Autodesk Inventor part; units mm, degrees
ref_plane "YZ Plane" through (0, 0, 0) normal (1, 0, 0) x (0, 1, 0)
ref_plane "XZ Plane" through (0, 0, 0) normal (0, 1, 0) x (-1, 0, 0)
ref_plane "XY Plane" through (0, 0, 0) normal (0, 0, 1) x (1, 0, 0)
sketch "Boceto1" plane through (0, 0, 0) normal (0, 1, 0) x (-1, 0, 0)
  circle A0 centre (0, 0) radius 26
  circle A1 centre (0, 0) radius 32
  line L0 (0, 40) -> (32, 40)
  line L1 (32, 40) -> (32, -40)
  line L2 (32, -40) -> (0, -40)
  line L3 (0, -40) -> (0, 40)
  dimension "d0" = 52
  dimension "d1" = 64
  dimension "d2" = 40
  dimension "d3" = 80
  dimension "d4" = 32
  dimension "d5" = 32
extrude "Extrusión1" add sketch "Boceto1" along normal blind 67
sketch "Boceto2" plane through (0, 67, 0) normal (0, 1, 0) x (1, 0, 0)
  circle A0 centre (0, 0) radius 26
  dimension "d8" = 52
hole "Agujero1" at (0, 67, 0) direction (0, -1, 0) diameter 52 depth 60
sketch "Boceto3" plane through (0, 0, 0) normal (0, -1, 0) x (1, 0, 0)
  circle A0 centre (0, 0) radius 13
  dimension "d16" = 26
hole "Agujero2" at (0, 0, 0) direction (0, 1, 0) diameter 26 depth 60
sketch "Boceto4" plane through (0, 0, 0) normal (0, -1, 0) x (1, 0, 0)
  circle A0 centre (0, 0) radius 17.75
  circle A1 centre (17.75, 0) radius 2
  circle A2 centre (0, -17.75) radius 2
  circle A3 centre (-17.75, 0) radius 2
  circle A4 centre (0, 17.75) radius 2
  dimension "d24" = 35.5
  dimension "d25" = 4
  dimension "d26" = 4
  dimension "d27" = 4
  dimension "d28" = 4
hole "Agujero3" at (17.75, 0, 0) at (0, 0, -17.75) at (-17.75, 0, 0) at (0, 0, 17.75) direction (0, 1, 0) diameter 4 depth 60
sketch "Boceto5" plane through (0, 67, 0) normal (0, 1, 0) x (1, 0, 0)
  point P0 (0, 0)
  point P1 (0, 0)
hole "Agujero4" at (0, 67, 0) direction (0, -1, 0) diameter 200 depth 7
sketch "Boceto6" plane through (-32, 0, -40) normal (-1, 0, 0) x (0, 0, 1)
  line L0 (4, 12.5) -> (76, 12.5)
  line L1 (76, 12.5) -> (76, 47.5)
  line L2 (76, 47.5) -> (4, 47.5)
  line L3 (4, 47.5) -> (4, 12.5)
  line L4 (4, 12.5) -> (76, 47.5) construction
  line L5 (76, 12.5) -> (4, 47.5) construction
  line L6 (80, 0) -> (80, 60)
  line L7 (80, 60) -> (0, 60)
  circle A0 centre (4, 47.5) radius 2
  circle A1 centre (76, 47.5) radius 2
  circle A2 centre (76, 12.5) radius 2
  circle A3 centre (4, 12.5) radius 2
  point P0 (40, 0)
  point P1 (40, 30)
  dimension "d43" = 35
  dimension "d44" = 40
  dimension "d45" = 30
  dimension "d46" = 72
  dimension "d47" = 4
  dimension "d48" = 4
  dimension "d49" = 4
  dimension "d50" = 4
hole "Agujero5" at (-32, 47.5, -36) at (-32, 12.5, -36) at (-32, 12.5, 36) at (-32, 47.5, 36) direction (1, 0, 0) diameter 4 depth 32
properties part number "BracketHusillo"
CAD build for the part. Positions are in the model's coordinates, mm. A direction names the side the tool comes from. Coordinates: 2 decimals unless noted, no trailing zeros. Write each loop counter-clockwise with the first axis right and the second up, starting at its lowest first coordinate (ties: lowest second). Pieces come first, ordered by that corner, then holes.
(1) Cut at D-D, the plane x = 7.5. List the corners of the cut face in (y, z), and give its area (3 significant figures).
(2) 3-axis set-ups, long thin cutter, end or side, ignore diameter. For faces 1 (the face through (-12, 7, -6)), 2 (the face through (-16, 30, -40)), 3 (the face through (0, 30, -36)): which of +Z, -Z, +X, -X, +Y, -Y reach the whole face in a straight line?
(3) Cut at C-C, the plane z = 36. List the corners of the cut face in (x, y).
(4) Cut at A-A, the plane y = 47.5. List the corners of the cut face in (x, z), and give its area (3 significant figures).
(5) Cut at B-B, the plane x = -5.5. List the corners of the cut face in (y, z), and give its area (3 significant figures).
(6) Drill centre lines: probe 1 along Y at (x, z) = (-11, 36); probe 2 along X at (y, z) = (2, 0); probe 3 along Z at (x, y) = (-17, 12). Where is each one in solid material? Low to high.
(7) Flat gauge pins, fed straight in: pin 1 (2 mm diameter, centred on y = 16, z = -6.5, fed in from +X); pin 2 (3 mm diameter, centred on x = 21.5, y = 22, fed in from -Z); pin 3 (1.5 mm diameter, centred on y = 12.5, z = -13.5, fed in from +X). Where does each tip first touch, or does it go through?
(8) Two-plate mould, pull along Z, no slides. Class faces 4 (the face through (0, 30, 36)), 5 (the face through (7.91, 3.549, 10.316)), 6 (the face through (-16, 30, 40)): +Z half, -Z half, draft (parallel to the pull), parting line (faces both ways), or undercut.
Geometry says:
1. outline: (0, -31.11) - (60, -31.11) - (60, -24.89) - (7, -24.89) - (7, -10.62) - (0, -10.62) - close; (0, 10.62) - (7, 10.62) - (7, 24.89) - (60, 24.89) - (60, 31.11) - (0, 31.11) - close
1. area: 946 mm2
2. face 1: +Y
2. face 2: -Z, +X, -X, +Y, -Y
2. face 3: -Z, +X, +Y, -Y
3. outline: (-32, 0) - (0, 0) - (0, 10.5) - (-32, 10.5) - close; (-32, 14.5) - (0, 14.5) - (0, 45.5) - (-32, 45.5) - close; (-32, 49.5) - (0, 49.5) - (0, 60) - (-32, 60) - close
4. outline: (-32, -40) - (0, -40) - (0, -38) - (-32, -38) - close; (-32, -34) - (0, -34) - (0, -32) arc R32 ccw to (0, 32) - (0, 34) - (-32, 34) - close; (-32, 38) - (0, 38) - (0, 40) - (-32, 40) - close; hole circle Ø52 at (0, 0)
4. area: 1,790 mm2
5. outline: (0, -40) - (60, -40) - (60, -25.41) - (7, -25.41) - (7, -11.78) - (0, -11.78) - close; (0, 11.78) - (7, 11.78) - (7, 25.41) - (60, 25.41) - (60, 40) - (0, 40) - close; hole circle Ø4 at (12.5, -36); hole circle Ø4 at (12.5, 36); hole circle Ø4 at (47.5, -36); hole circle Ø4 at (47.5, 36)
5. area: 1,890 mm2
6. probe 1: y = 0 to 10.5, 14.5 to 45.5, 49.5 to 60
6. probe 2: x = -32 to -19.75, -15.75 to -13, 13 to 15.75, 19.75 to 32
6. probe 3: z = -40 to -37.94, -34.06 to -19.67, 19.67 to 34.06, 37.94 to 40
7. pin 1: stops at x = 31.52
7. pin 2: stops at z = -24.98
7. pin 3: stops at x = 29.35
8. face 4: draft
8. face 5: undercut
8. face 6: +Z half
